Source: CAD feature listing. Evaluate the final solid. Frame: model axes, mm. A direction names the side the tool comes from. Give positions to 0.01 mm unless a question says otherwise; leave off trailing zeros. Write each loop counter-clockwise with the first axis right and the second up, starting at its lowest first coordinate (ties: lowest second). Pieces come first, ordered by that corner, then holes. Notation, with made-up numbers: (54.5, 67.5) -> (101.5, 67.5) arc R16 ccw to (101.5, 76.5) -> close; hole circle Ø9 at (88.5, 72). An arc over 180 degrees is marked (long way). Use one line per item in the form item = value. Start each with the question number.
(1) Cut plane C-C, the plane z = 21.5. Output: boundary loops of the cut face in (x, y), and give its area (3 significant figures).
(2) Cut plane B-B, the plane z = 30. Output: boundary loops of the cut face in (x, y), and give its area (3 significant figures).
(3) Cut plane A-A, the plane y = 0. Output: boundary loops of the cut face in (x, z).
(4) First-contact query: P1, Ø5, axis at x = 5.5, y = -6, coming from the -Z side; P2, Ø2, axis at y = 0, z = 11, coming from the +X side; P3, Ø6, axis at y = -4.5, z = 16.5, coming from the -X side. Flat tips, straight axial feed; report the tip coordinate or a pass-through.
(5) Cut plane D-D, the plane y = -5.25. Output: boundary loops of the cut face in (x, z), and give its area (3 significant figures).
(6) Set-up query: faces 1 (the face through (23, 0, 33)), 2 (the face through (0, 10, 20)), 3 (the face through (-23, 0, 33)). Return all of +Z, -Z, +X, -X, +Y, -Y with unobstructed straight access to the full face (end or side cutting, diameter ignored); none if empty.
(7) Material intervals for line 1 along X through (y, z) = (-0.5, 2), sorted ascending. Write a range as from..to.
from build123d import *

# Parameters (mm, degrees)
CROQUIS1_W              = 40
CROQUIS1_H              = 20
SALIENTE_EXTRUIR1_DEPTH = 40
CROQUIS2_R              = 3
SALIENTE_EXTRUIR2_DEPTH = 5.5


with BuildPart() as part:
    # Croquis1 → Saliente-Extruir1 (new body)
    with BuildSketch(Plane.XY):
        Rectangle(CROQUIS1_W, CROQUIS1_H)
    extrude(amount=SALIENTE_EXTRUIR1_DEPTH)

    # Croquis2 → Saliente-Extruir2 (add)
    with BuildSketch(Plane.ZY.offset(20)):
        with Locations(Location((30, 0, 0), (0, 0, 180))):
            Circle(CROQUIS2_R)
    saliente_extruir2 = extrude(amount=SALIENTE_EXTRUIR2_DEPTH)

    # Simetría1: Saliente-Extruir2 across plane
    add(saliente_extruir2.mirror(Plane(origin=(0, 0, 0), x_dir=(0, 0, 1), z_dir=(1, 0, 0))))


solid = part.part
Geometry says:
q1.outline = (-20, -10) -> (20, -10) -> (20, 10) -> (-20, 10) -> close
q1.area = 800 mm^2
q2.outline = (-25.5, -3) -> (-20, -3) -> (-20, -10) -> (20, -10) -> (20, -3) -> (25.5, -3) -> (25.5, 3) -> (20, 3) -> (20, 10) -> (-20, 10) -> (-20, 3) -> (-25.5, 3) -> close
q2.area = 866 mm^2
q3.outline = (-25.5, 27) -> (-20, 27) -> (-20, 0) -> (20, 0) -> (20, 27) -> (25.5, 27) -> (25.5, 33) -> (20, 33) -> (20, 40) -> (-20, 40) -> (-20, 33) -> (-25.5, 33) -> close
q4.P1 = 0
q4.P2 = 20
q4.P3 = -20
q5.outline = (-20, 0) -> (20, 0) -> (20, 40) -> (-20, 40) -> close
q5.area = 1,600 mm^2
q6.face_1 = +X
q6.face_2 = +Z, -Z, +X, -X, +Y
q6.face_3 = -X
q7.line_1 = -20..20
